Source: CAD feature listing. Evaluate the final solid. Frame: model axes, mm. Give positions to 0.01 mm unless a question says otherwise; leave off trailing zeros. Write each loop counter-clockwise with the first axis right and the second up, starting at its lowest first coordinate (ties: lowest second). Pieces come first, ordered by that corner, then holes. Notation, with made-up numbers: (-17, 33.25) -> (24, 33.25) arc R27 cw to (24, 57.25) -> close; hole circle Ø5 at (52.25, -10.5). An arc over 180 degrees is marked (long way). Write item = value, one per line.
from build123d import *

# Parameters (mm, degrees)
F_5MM_START          = 27
SKETCH_1_W           = 64
SKETCH_1_H           = 44
F_5MM_DEPTH          = 5
CUT_EXTRUDE_START    = 27
SKETCH_2_R           = 1.55
CUT_EXTRUDE_48_DEPTH = 5


with BuildPart() as part:
    # 草图1 → 模拟5mm车架_非整车底板模型 (new body)
    with BuildSketch(Plane.XY.offset(F_5MM_START)):
        Rectangle(SKETCH_1_W, SKETCH_1_H)
    extrude(amount=F_5MM_DEPTH)

    # 草图2 → 检具48孔距 (cut)
    with BuildSketch(Plane.XY.offset(CUT_EXTRUDE_START)):
        with Locations((-24, 0)):
            Circle(SKETCH_2_R)
        with Locations((24, 0)):
            Circle(SKETCH_2_R)
    extrude(amount=CUT_EXTRUDE_48_DEPTH, mode=Mode.SUBTRACT)


solid = part.part
1) Cut plane A-A (y = 0). Return the cut outline in (x, z).
Computed:
outline = (-32, 27) -> (-25.55, 27) -> (-25.55, 32) -> (-32, 32) -> close; (-22.45, 27) -> (22.45, 27) -> (22.45, 32) -> (-22.45, 32) -> close; (25.55, 27) -> (32, 27) -> (32, 32) -> (25.55, 32) -> close
2) Material intervals for L1, parallel to Y at x = 24, z = 29.9; L2, parallel to Y at x = -23, z = 27.85, sorted ascending.
Computed:
L1 = -22 to -1.55, 1.55 to 22
L2 = -22 to -1.18, 1.18 to 22
3) Cut plane B-B (x = -24). Return the cut outline in (y, z), then the cut area to 4 significant figures.
Computed:
outline = (-22, 27) -> (-1.55, 27) -> (-1.55, 32) -> (-22, 32) -> close; (1.55, 27) -> (22, 27) -> (22, 32) -> (1.55, 32) -> close
area = 204.5 mm²
4) Draft query along Y for faces 1 (the flat face through (0, 22, 29)), 2 (the cylindrical face through (25.432, -0.594, 29.465)), 3 (the cylindrical face through (-22.568, -0.594, 29.465)), 4 (the flat face through (-32, 0, 29)). Return one class per face: pulls with the +Y half, pulls with the -Y half, needs draft (parallel to the pull), parting line crosses it, or undercut.
Computed:
face_1 = pulls with the +Y half
face_2 = undercut
face_3 = undercut
face_4 = needs draft
